Input: dimensioned drawing with shaded views. Units: mm. Origin: part minimum x, y, z. A direction names the side the tool comes from. Round coordinates to 2 decimals unless told otherwise and drop trailing zeros. Order: outer loops, then holes, each group sorted by start corner. A loop starts at its lowest first (then second) coordinate and runs counter-clockwise, first axis right, second up. Notation, with made-up numbers: (33.5, 77.25) - (58.5, 77.25) arc R16 cw to (58.5, 96.25) - close; hole circle Ø5 at (72.25, 85.25). An arc over 180 degrees is marked (long way). Return JSON: item names as keys, results as strings. Group by question number.
1) Contact query for a flat-ended pin moving along its axis: P1, Ø1, axis at x = 863.5, y = 61.5, coming from the +Z side. Output: stop coordinate, or through.
2) Ray query, line 1 (Z direction, x = 630, y = 147); line 2 (X direction, y = 356.5, z = 618); line 3 (Z direction, x = 283.5, y = 166). Return the intervals inside material, ascending. Write a range as from..to.
3) Access query for the marked faces 1 and 2. Directions: +Z, -Z, +X, -X, +Y, -Y. A direction counts if a zero-diameter tool reaches every point of the face in a straight line with its end or side. Return the directions, or none.
4) Section B-B, the plane y = 304.8. Return loops of the section in (x, z), plus the area to 3 significant figures.
5) Section C-C, the plane x = 1084. Return loops of the section in (y, z), plus the area to 3 significant figures.
6) Section A-A, the plane x = 304.8. Return loops of the section in (y, z).
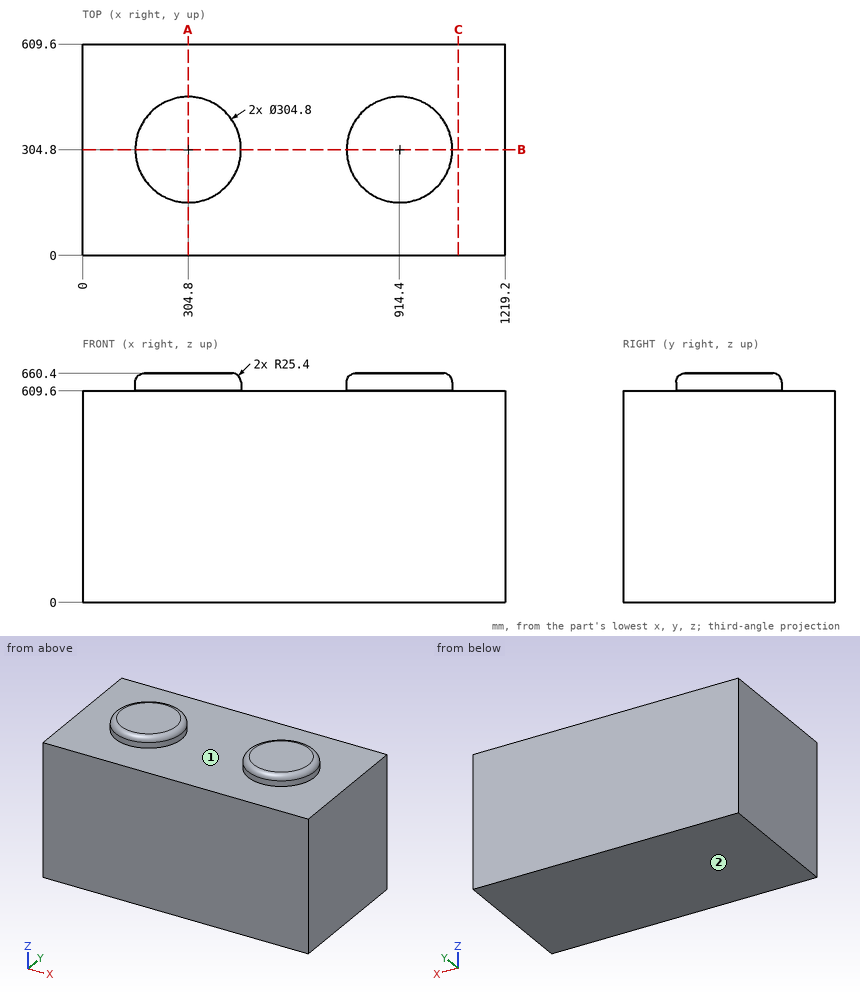
Geometry check:
{
 "1": {"P1": "z = 609.6"},
 "2": {"line 1": "0..609.6", "line 2": "161.44..448.16, 771.04..1057.76", "line 3": "0..656.56"},
 "3": {"face 1": "+Z", "face 2": "-Z, +X, -X, +Y, -Y"},
 "4": {"outline": "(0, 0) - (1219.2, 0) - (1219.2, 609.6) - (1066.8, 609.6) - (1066.8, 635) arc R25.4 ccw to (1041.4, 660.4) - (787.4, 660.4) arc R25.4 ccw to (762, 635) - (762, 609.6) - (457.2, 609.6) - (457.2, 635) arc R25.4 ccw to (431.8, 660.4) - (177.8, 660.4) arc R25.4 ccw to (152.4, 635) - (152.4, 609.6) - (0, 609.6) - close", "area": "774,000 mm2"},
 "5": {"outline": "(0, 0) - (609.6, 0) - (609.6, 609.6) - (0, 609.6) - close", "area": "372,000 mm2"},
 "6": {"outline": "(0, 0) - (609.6, 0) - (609.6, 609.6) - (457.2, 609.6) - (457.2, 635) arc R25.4 ccw to (431.8, 660.4) - (177.8, 660.4) arc R25.4 ccw to (152.4, 635) - (152.4, 609.6) - (0, 609.6) - close"}
}
